from build123d import *

# Parameters (mm, degrees)
F0_W          = 1524
F0_H          = 101.6
F1_DEPTH      = 25.4
F1_DEPTH_BACK = 25.4
F2_W          = 25.4
F2_H          = 76.2
F3_DEPTH      = 76.2
F4_W          = 25.4
F4_H          = 76.2
F5_DEPTH      = 76.2


with BuildPart() as f1:
    # F0 (on Right) → F1 (new body, two sides)
    with BuildSketch(Plane.YZ) as f1_sk:
        Rectangle(F0_W, F0_H)
    extrude(amount=F1_DEPTH)
    extrude(f1_sk.sketch, amount=-F1_DEPTH_BACK)

    # F2 (on face) → F3 (join)
    with BuildSketch(Plane(origin=(0, 762, 0), x_dir=(-1, 0, 0), z_dir=(0, 1, 0))):
        Rectangle(F2_W, F2_H)
    extrude(amount=F3_DEPTH)

    # F4 (on face) → F5 (join)
    with BuildSketch(Plane.XZ.offset(762)):
        Rectangle(F4_W, F4_H)
    extrude(amount=F5_DEPTH)


solid = f1.part
Work out the finished part from the listing and answer in its coordinate system (mm). A direction names the side the tool comes from. Coordinates: 2 decimals unless noted, no trailing zeros. Write each loop counter-clockwise with the first axis right and the second up, starting at its lowest first coordinate (ties: lowest second). Pieces come first, ordered by that corner, then holes. Notation, with made-up numbers: M -3.5,35 L 18.5,35 A8 cw 18.5,50 Z; hole C 38,16 d7. An arc over 180 degrees is marked long. Write item = value, one per line.
1. Flat-ended cylindrical pins translate along their axes: pin 1 (7.5 mm diameter, centred on x = 4, y = 810.5, fed in from -Z); pin 2 (3 mm diameter, centred on x = 18, z = -24.5, fed in from -Y). Find the tip coordinate at first contact, or state that the pin passes through.
Solution:
pin_1 = -38.1
pin_2 = -762
2. The part is cut by section B-B (x = 2). Determine the outline of the cut face in (y, z), then the cut area to 3 significant figures.
Solution:
outline = M -838.2,-38.1 L -762,-38.1 L -762,-50.8 L 762,-50.8 L 762,-38.1 L 838.2,-38.1 L 838.2,38.1 L 762,38.1 L 762,50.8 L -762,50.8 L -762,38.1 L -838.2,38.1 Z
area = 166,000 mm2
3. The part is cut by section A-A (z = 11). Determine the outline of the cut face in (x, y), then the cut area to 3 significant figures.
Solution:
outline = M -25.4,-762 L -12.7,-762 L -12.7,-838.2 L 12.7,-838.2 L 12.7,-762 L 25.4,-762 L 25.4,762 L 12.7,762 L 12.7,838.2 L -12.7,838.2 L -12.7,762 L -25.4,762 Z
area = 81,300 mm2
4. A straight line is drawn through the part: line 1 (Y direction, x = -6, z = -43). Find the intervals that lie inside material, in ascending order. Write a range as from..to.
Solution:
line_1 = -762..762
5. For faces 1 (the face through (-12.7, -800, -1)), 2 (the face through (12.7, 800, -1)), 3 (the face through (12.7, -800, -1)), 4 (the face through (0, 800, -38.1)), determine the directions among +Z, -Z, +X, -X, +Y, -Y from which every point of the face is accessible in a straight line to the end or side of a thin tool.
Solution:
face_1 = +Z, -Z, -X, -Y
face_2 = +Z, -Z, +X, +Y
face_3 = +Z, -Z, +X, -Y
face_4 = -Z, +X, -X, +Y
